Check sheet for the modelled part. Datum: model origin and axes. Units: mm. Round coordinates to 2 decimals unless told otherwise and drop trailing zeros. Use one line per item in the form item = value. Start each with the question number.
(1) Sectioned sample at A-A (z = 26.5). State how many separate pieces and enclosed holes the cut face has, and give its area (3 significant figures).
(2) Go/stop test with flat-tipped pins: pin 1 (4 mm diameter, centred on x = 0, z = 186.5, fed in from -Y); pin 2 (2 mm diameter, centred on x = -2.5, z = 155, fed in from -Y); pin 3 (1 mm diameter, centred on x = -5.5, z = 96.5, fed in from -Y). Record where each tip stops, or that it passes through.
(3) Material ranges on probe 1 along X at (y, z) = (5.75, 245); probe 2 along X at (y, z) = (-4.5, 258.5); probe 3 along Y at (x, z) = (-5.25, 170), recorded low to high. Write a range as [from, to].
from build123d import *

# Parameters (mm, degrees)
BOSS_EXTRU_1_DEPTH = 300


with BuildPart() as part:
    # Esquisse1 → Boss.-Extru.1 (new body)
    with BuildSketch(Plane.XY):
        with BuildLine():
            Line((-2.277781394, 7.764570671), (-7.068879094, 7.764570671))
            ThreePointArc((-7.068879094, 7.764570671), (-8.417278819, 7.241668562), (-9.060597485, 5.946388851))
            ThreePointArc((-9.060597485, 5.946388851), (-9.659264868, 2.58818977), (-10.819903246, -0.619429637))
            ThreePointArc((-10.819903246, -0.619429637), (-10.910412794, -2.062834106), (-10.00411543, -3.18988048))
            Line((-10.00411543, -3.18988048), (-5.834093414, -5.597443814))
            ThreePointArc((-5.834093414, -5.597443814), (-5.236709364, -5.662062276), (-4.7628449, -5.292609007))
            Line((-4.7628449, -5.292609007), (-4.412844891, -4.68639123))
            ThreePointArc((-4.412844891, -4.68639123), (-4.382874764, -4.458745516), (-4.522652512, -4.276583608))
            Line((-4.522652512, -4.276583608), (-6.356537861, -3.217789408))
            ThreePointArc((-6.356537861, -3.217789408), (-6.765622267, -2.388248296), (-6.155776036, -1.692851946))
            Line((-6.155776036, -1.692851946), (-3.081802459, -0.869183204))
            ThreePointArc((-3.081802459, -0.869183204), (-1.913766747, -0.792626099), (-0.805345324, -1.168884471))
            Line((-0.805345324, -1.168884471), (1.159782546, -2.303451576))
            ThreePointArc((1.159782546, -2.303451576), (2.039842566, -3.075243499), (2.557560023, -4.125070649))
            Line((2.557560023, -4.125070649), (3.381228766, -7.199044225))
            ThreePointArc((3.381228766, -7.199044225), (3.083920975, -8.074884735), (2.160975089, -8.135377804))
            Line((2.160975089, -8.135377804), (0.32708974, -7.076583604))
            ThreePointArc((0.32708974, -7.076583604), (0.099444026, -7.046613477), (-0.082717881, -7.186391225))
            Line((-0.082717881, -7.186391225), (-0.432717881, -7.792609008))
            ThreePointArc((-0.432717881, -7.792609008), (-0.515741566, -8.3877143), (-0.161088322, -8.872754831))
            Line((-0.161088322, -8.872754831), (3.885572059, -11.209095291))
            ThreePointArc((3.885572059, -11.209095291), (5.453886583, -11.394599855), (6.667853821, -10.384497912))
            ThreePointArc((6.667853821, -10.384497912), (9.659251661, -2.588191136), (10.966778527, 5.659307508))
            ThreePointArc((10.966778527, 5.659307508), (10.420503025, 7.141065072), (8.969550516, 7.764570662))
            Line((8.969550516, 7.764570662), (4.322218596, 7.764570662))
            ThreePointArc((4.322218596, 7.764570662), (3.756533171, 7.530256087), (3.522218596, 6.964570662))
            Line((3.522218596, 6.964570662), (3.522218596, 6.264570662))
            ThreePointArc((3.522218596, 6.264570662), (3.610086561, 6.052438628), (3.822218596, 5.964570662))
            Line((3.822218596, 5.964570662), (5.939806996, 5.964570662))
            ThreePointArc((5.939806996, 5.964570662), (6.708855039, 5.450709188), (6.528410886, 4.543555168))
            Line((6.528410886, 4.543555168), (4.278106046, 2.293250328))
            ThreePointArc((4.278106046, 2.293250328), (3.304835999, 1.642932074), (2.156785702, 1.414570672))
            Line((2.156785702, 1.414570672), (-0.112348508, 1.414570672))
            ThreePointArc((-0.112348508, 1.414570672), (-1.260398803, 1.642932074), (-2.233668848, 2.293250327))
            Line((-2.233668848, 2.293250327), (-4.483973688, 4.543555167))
            ThreePointArc((-4.483973688, 4.543555167), (-4.664417843, 5.450709193), (-3.895369794, 5.964570671))
            Line((-3.895369794, 5.964570671), (-1.777781394, 5.964570671))
            ThreePointArc((-1.777781394, 5.964570671), (-1.565649359, 6.052438637), (-1.477781394, 6.264570671))
            Line((-1.477781394, 6.264570671), (-1.477781394, 6.964570671))
            ThreePointArc((-1.477781394, 6.964570671), (-1.712095969, 7.530256096), (-2.277781394, 7.764570671))
        make_face()
        with BuildLine():
            Line((-7.323961592, 5.240984459), (-7.661560194, 3.19617001))
            ThreePointArc((-7.661560194, 3.19617001), (-7.657816372, 3.097611471), (-7.607424532, 3.012826659))
            Line((-7.607424532, 3.012826659), (-7.57849861, 2.983900741))
            ThreePointArc((-7.57849861, 2.983900741), (-7.520213219, 2.853306067), (-7.56403866, 2.717175664))
            ThreePointArc((-7.56403866, 2.717175664), (-7.87179554, 2.110471478), (-7.908622362, 1.431171801))
            ThreePointArc((-7.908622362, 1.431171801), (-7.938733618, 1.291366699), (-8.05450758, 1.20741109))
            Line((-8.05450758, 1.20741109), (-8.094021121, 1.196823472))
            ThreePointArc((-8.094021121, 1.196823472), (-8.180054139, 1.148593589), (-8.23257565, 1.0651113))
            Line((-8.23257565, 1.0651113), (-8.962613913, -0.874549263))
            ThreePointArc((-8.962613913, -0.874549263), (-8.771314591, -1.392312789), (-8.244983453, -1.226029799))
            ThreePointArc((-8.244983453, -1.226029799), (-7.559869341, -0.421536961), (-6.6135889, 0.048721903))
            ThreePointArc((-6.6135889, 0.048721903), (-6.572819287, 0.055124525), (-6.531603527, 0.053023068))
            ThreePointArc((-6.531603527, 0.053023068), (-5.816110839, 0.099392966), (-5.18783842, 0.444869046))
            ThreePointArc((-5.18783842, 0.444869046), (-5.101288158, 0.489475582), (-5.003931638, 0.487926814))
            Line((-5.003931638, 0.487926814), (-4.707356797, 0.408459826))
            ThreePointArc((-4.707356797, 0.408459826), (-4.585051414, 0.414498293), (-4.489190426, 0.490693704))
            ThreePointArc((-4.489190426, 0.490693704), (-4.201277401, 1.126959114), (-4.132484687, 1.821937635))
            ThreePointArc((-4.132484687, 1.821937635), (-4.177405034, 1.935855289), (-4.280305369, 2.002237445))
            Line((-4.280305369, 2.002237445), (-4.576880211, 2.081704429))
            ThreePointArc((-4.576880211, 2.081704429), (-4.661967815, 2.129041419), (-4.714619271, 2.210946946))
            ThreePointArc((-4.714619271, 2.210946946), (-5.085981109, 2.82427422), (-5.682431007, 3.222178075))
            ThreePointArc((-5.682431007, 3.222178075), (-5.719175628, 3.240966039), (-5.751281836, 3.266895679))
            ThreePointArc((-5.751281836, 3.266895679), (-6.335655302, 4.147292021), (-6.526735107, 5.186560309))
            ThreePointArc((-6.526735107, 5.186560309), (-6.899409756, 5.593731171), (-7.323961592, 5.240984459))
        make_face(mode=Mode.SUBTRACT)
        with BuildLine():
            Line((4.039005672, -0.226915238), (3.742430831, -0.147448251))
            ThreePointArc((3.742430831, -0.147448251), (3.620125447, -0.153486718), (3.524264457, -0.22968213))
            ThreePointArc((3.524264457, -0.22968213), (3.236351435, -0.865947537), (3.167558721, -1.560926054))
            ThreePointArc((3.167558721, -1.560926054), (3.212479068, -1.674843705), (3.3153794, -1.74122586))
            Line((3.3153794, -1.74122586), (3.611954241, -1.820692845))
            ThreePointArc((3.611954241, -1.820692845), (3.697041845, -1.868029834), (3.749693301, -1.949935361))
            ThreePointArc((3.749693301, -1.949935361), (4.120587374, -2.562773684), (4.716243148, -2.960677472))
            ThreePointArc((4.716243148, -2.960677472), (4.822262289, -3.056657136), (4.837082998, -3.198898132))
            Line((4.837082998, -3.198898132), (4.519637838, -4.383619602))
            ThreePointArc((4.519637838, -4.383619602), (4.512823004, -4.435383412), (4.519637838, -4.487147222))
            Line((4.519637838, -4.487147222), (5.227723978, -7.129760649))
            ThreePointArc((5.227723978, -7.129760649), (5.675553803, -7.499115267), (6.170739428, -7.196186922))
            Line((6.170739428, -7.196186922), (7.455923223, -3.717453783))
            ThreePointArc((7.455923223, -3.717453783), (7.459439401, -3.609785311), (7.406594848, -3.515911372))
            Line((7.406594848, -3.515911372), (6.613572648, -2.722889172))
            ThreePointArc((6.613572648, -2.722889172), (6.555287263, -2.592294501), (6.599112704, -2.456164105))
            ThreePointArc((6.599112704, -2.456164105), (6.906869584, -1.849459918), (6.943696406, -1.170160238))
            ThreePointArc((6.943696406, -1.170160238), (6.973807663, -1.030355137), (7.089581623, -0.946399529))
            Line((7.089581623, -0.946399529), (8.172870105, -0.656133266))
            ThreePointArc((8.172870105, -0.656133266), (8.2655718, -0.601258323), (8.316360933, -0.506256599))
            Line((8.316360933, -0.506256599), (8.942725678, 3.149006571))
            ThreePointArc((8.942725678, 3.149006571), (8.665346523, 3.658943048), (8.092837193, 3.56298747))
            Line((8.092837193, 3.56298747), (6.158309903, 1.62846018))
            ThreePointArc((6.158309903, 1.62846018), (6.126526177, 1.587038823), (6.106546092, 1.53880263))
            Line((6.106546092, 1.53880263), (5.789100936, 0.35408116))
            ThreePointArc((5.789100936, 0.35408116), (5.705145325, 0.238307201), (5.565340223, 0.208195951))
            ThreePointArc((5.565340223, 0.208195951), (4.850535301, 0.161429048), (4.222912453, -0.18385747))
            ThreePointArc((4.222912453, -0.18385747), (4.136362192, -0.228464006), (4.039005672, -0.226915238))
        make_face(mode=Mode.SUBTRACT)
    extrude(amount=BOSS_EXTRU_1_DEPTH)


solid = part.part
Checks:
q1.separate_pieces = 1
q1.enclosed_holes = 2
q1.area = 169 mm2
q2.pin_1 = -10.12
q2.pin_2 = -0.98
q2.pin_3 = -5.69
q3.probe_1 = [-9.08, -4.45], [6.5, 10.97]
q3.probe_2 = [-7.73, -4.37], [2.66, 4.52], [7.17, 9.1]
q3.probe_3 = [-5.67, -3.86], [-1.45, 0.39], [2.97, 7.76]
